For this review, use the dimensioned drawing (mm, ordinates from the lowest corner) and the shaded views. Round coordinates to 2 decimals unless told otherwise and drop trailing zeros. Write each loop counter-clockwise with the first axis right and the second up, starting at its lowest first coordinate (ties: lowest second). Pieces come first, ordered by that corner, then holes. Notation, with made-up numbers: M 42.25,67.5 L 50.25,67.5 A24 ccw 50.25,88.5 Z; hole C 84.25,26.5 d8. An arc over 180 degrees is marked long. Write each question's results on one line, items separated by ' | '. Start each with the question number.
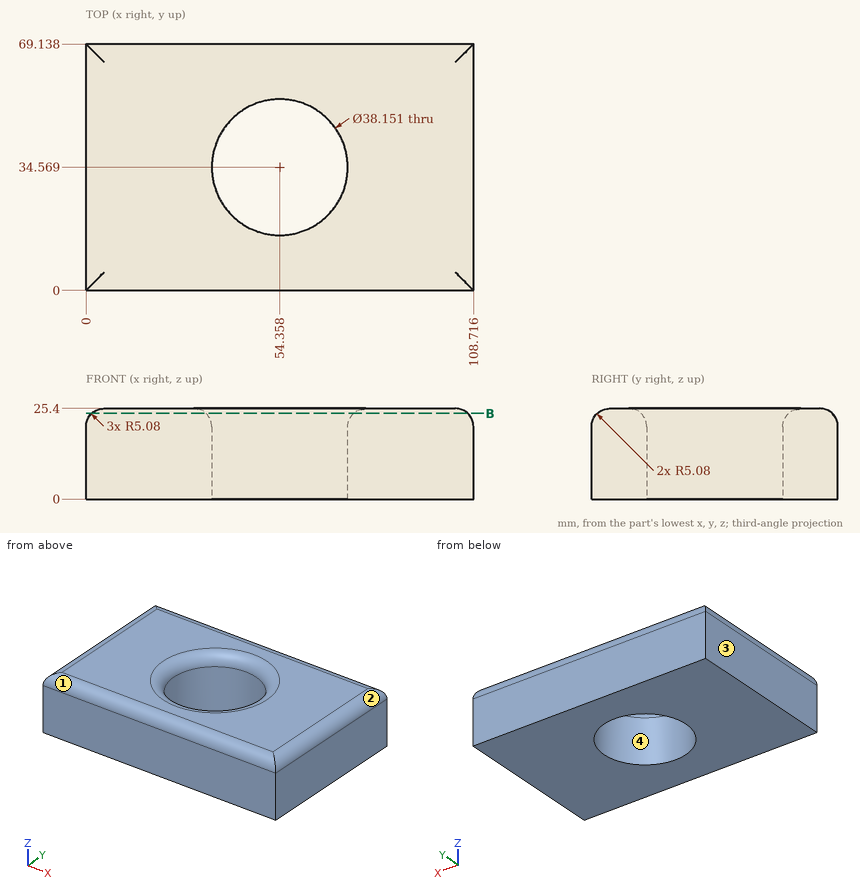
Item 1: Mouldability with a two-part tool opening along X and no side actions: class the marked faces 1, 2, 3 and 4 as pulls with the +X half, pulls with the -X half, needs draft (parallel to the pull), parting line crosses it, or undercut.
Item 2: For probe 1 along Y at (x, z) = (40, 7.25); probe 2 along Y at (x, z) = (62.5, 13); probe 3 along X at (y, z) = (38.5, 6.5) (1 decimal), list the stretches that pass through material, from the lowest coordinate up.
Item 3: We need section B-B on z = 24. State the section outline as (x, y) points.
Item 4: Insertion check: P1, Ø10, axis at y = 37.5, z = 6, coming from the -X side; P2, Ø23, axis at x = 54.36, y = 34.57, coming from the -Z side. Each pin has a flat end and moves straight along its axis. Give the tip position at first contact, or say it passes through.
Numbers:
1) face 1: needs draft | face 2: pulls with the +X half | face 3: pulls with the -X half | face 4: undercut
2) probe 1: y = 0 to 22.01, 47.13 to 69.14 | probe 2: y = 0 to 17.32, 51.82 to 69.14 | probe 3: x = 0 to 35.7, 73 to 108.7
3) outline: M 1.58,1.58 L 107.14,1.58 L 107.14,67.56 L 1.58,67.56 Z; hole C 54.36,34.57 d41.31
4) P1: stops at x = 0 | P2: passes through
